from build123d import *

# Parameters (mm, degrees)
BOSS_EXTRUDE1_DEPTH = 3.15
SKETCH2_R           = 1.625
CUT_EXTRUDE1_DEPTH  = 2


with BuildPart() as part:
    # Sketch1 → Boss-Extrude1 (new body)
    with BuildSketch(Plane(origin=(0, 0, 0), x_dir=(1, 0, 0), z_dir=(0, 1, 0))):
        with BuildLine():
            Line((-17.971705397, 32.627906846), (-13.729256498, 25.279769804))
            ThreePointArc((-13.729256498, 25.279769804), (0, 28.767329478), (13.729256498, 25.279769804))
            Line((13.729256498, 25.279769804), (17.971705397, 32.627906846))
            ThreePointArc((17.971705397, 32.627906846), (0, 37.25), (-17.971705397, 32.627906846))
        make_face()
    extrude(amount=BOSS_EXTRUDE1_DEPTH)

    # Sketch2 → Cut-Extrude1 (cut)
    with BuildSketch(Plane.XZ):
        with Locations(Location((0, -33.008664739, 0), (0, 0, 270))):
            Circle(SKETCH2_R)
    extrude(amount=-CUT_EXTRUDE1_DEPTH, mode=Mode.SUBTRACT)


solid = part.part
The listing builds one solid part. Answer for the finished solid, in the listing's coordinates (mm). Give positions to 0.01 mm unless a question says otherwise; leave off trailing zeros. Write each loop counter-clockwise with the first axis right and the second up, starting at its lowest first coordinate (ties: lowest second). Pieces come first, ordered by that corner, then holes. Notation, with made-up numbers: (23.25, 58) - (54.25, 58) arc R23 ccw to (54.25, 85) - close; hole circle Ø10 at (0.5, -30.75). An arc over 180 degrees is marked (long way). One line per question, with ' | ' between items. Start each with the question number.
1. Determine the mould class of faces 1 (the face through (-15.88, 1.553, -29.005)), 2 (the face through (0, 0, -31)), 3 (the face through (0, 2, -33)), 4 (the face through (0.49, 0.99, -34.56)) for opening direction X: +X half, -X half, draft (parallel to the pull), parting line (faces both ways), or undercut.
2. Given P1, Ø1, axis at y = 2.5, z = -27.5, coming from the +X side, flat-ended and moving along its own axis, determine where the tip first touches the part or whether it passes through.
3. Section B-B, the plane x = 0 is taken. Determine the outline of the cut face in (y, z), then the cut area to 3 significant figures.
4. Section D-D, the plane x = 7.5 is taken. Determine the outline of the cut face in (y, z), then the cut area to 3 significant figures.
5. Section C-C, the plane z = -32 is taken. Determine the outline of the cut face in (x, y), then the cut area to 3 significant figures.
6. Section A-A, the plane z = -26 is taken. Determine the outline of the cut face in (x, y), then the cut area to 3 significant figures.
7. Straight lines are drawn through the part: line 1 (X direction, y = 0.25, z = -34); line 2 (X direction, y = 1.25, z = -33.75); line 3 (Z direction, x = -2, y = 0.4). For each, find the intervals that lie inside material, in ascending order.
Result:
1) face 1: -X half | face 2: draft | face 3: undercut | face 4: undercut
2) P1: stops at x = 15.3
3) outline: (0, -37.25) - (3.15, -37.25) - (3.15, -28.77) - (0, -28.77) - (0, -31.38) - (2, -31.38) - (2, -34.63) - (0, -34.63) - close | area: 20.2 mm2
4) outline: (0, -36.49) - (3.15, -36.49) - (3.15, -27.77) - (0, -27.77) - close | area: 27.5 mm2
5) outline: (-17.61, 0) - (-1.27, 0) - (-1.27, 2) - (1.27, 2) - (1.27, 0) - (17.61, 0) - (17.61, 3.15) - (-17.61, 3.15) - close | area: 106 mm2
6) outline: (-14.15, 0) - (-12.31, 0) - (-12.31, 3.15) - (-14.15, 3.15) - close; (12.31, 0) - (14.15, 0) - (14.15, 3.15) - (12.31, 3.15) - close | area: 11.6 mm2
7) line 1: x = -15.22 to -1.29, 1.29 to 15.22 | line 2: x = -15.76 to -1.45, 1.45 to 15.76 | line 3: z = -37.2 to -28.7
